Check sheet for the modelled part. Datum: model origin and axes. Units: mm. Face numbers are marked on the shaded views. A direction names the side the tool comes from. Give positions to 0.01 mm unless a question says otherwise; leave off trailing zeros. Order: outer loops, then holes, each group sorted by start corner. A loop starts at its lowest first (then second) coordinate and runs counter-clockwise, first axis right, second up. Notation, with made-up numbers: (18.5, -18.75) -> (69.5, -18.75) arc R10 cw to (69.5, -10.75) -> close; hole circle Ø9 at (58, 17). An arc over 180 degrees is marked (long way). Write each question's results on one line, items separated by ' | '.
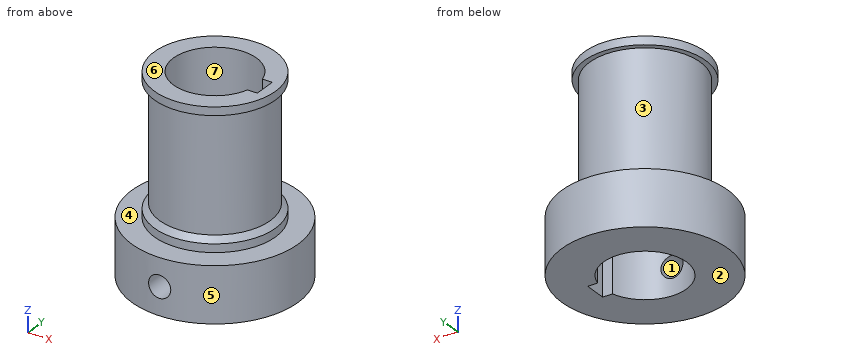
from build123d import *

# Parameters (mm, degrees)
F0_R      = 30
F1_DEPTH  = 20
F3_R      = 21.9
F4_DEPTH  = 3
F6_R      = 21.9
F7_DEPTH  = 2
F9_R      = 20
F10_DEPTH = 42
F11_SIZE2 = 1.99999
F11_SIZE  = 1.89999
F12_R     = 21.9
F13_DEPTH = 3
F15_DEPTH = 78
F16_R     = 4
F17_DEPTH = 45


# Not quite as in the source:
# - a fillet or chamfer is up to 0.001 mm smaller than in the source, because OpenCascade refuses the exact size


with BuildPart() as f1:
    # F0 (on Top) → F1 (new body)
    with BuildSketch(Plane.XY):
        Circle(F0_R)
    extrude(amount=F1_DEPTH)

    # F3 (on offset) → F4 (join)
    with BuildSketch(Plane.XY.offset(20)):
        Circle(F3_R)
    extrude(amount=F4_DEPTH)

    # F6 (on offset) → F7 (join)
    with BuildSketch(Plane.XY.offset(23)):
        Circle(F6_R)
    extrude(amount=F7_DEPTH)

    # F9 (on offset) → F10 (join)
    with BuildSketch(Plane.XY.offset(25)):
        Circle(F9_R)
    extrude(amount=F10_DEPTH)

    # F11 (size 1.9 and 2 in the source; OpenCascade refuses exactly that, so slightly less here)
    f11_edges = [f1.edges().sort_by_distance(p)[0] for p in [
        (-21.9, 0, 25),
    ]]
    f11_side = f1.faces().sort_by_distance((-21.280574, 0, 25))[0]
    chamfer(f11_edges, length=F11_SIZE, length2=F11_SIZE2, reference=f11_side)

    # F12 (on face) → F13 (join)
    with BuildSketch(Plane.XY.offset(67)):
        Circle(F12_R)
    extrude(amount=F13_DEPTH)

    # F14 (on face) → F15 (cut)
    with BuildSketch(Plane.XY.offset(70)):
        with BuildLine():
            Line((18, 4), (14.4568322948, 4))
            ThreePointArc((14.4568322948, 4), (-15, 0), (14.4568322948, -4))
            Line((14.4568322948, -4), (18, -4))
            Line((18, -4), (18, 0))
            Line((18, 0), (18, 4))
        make_face()
    extrude(amount=-F15_DEPTH, mode=Mode.SUBTRACT)

    # F16 (on Front) → F17 (cut)
    with BuildSketch(Plane.XZ):
        with Locations((0, 10)):
            Circle(F16_R)
    extrude(amount=F17_DEPTH, mode=Mode.SUBTRACT)


solid = f1.part
1. Gauge pin test, flat ends, axial feed: pin 1 Ø1.8 at (x, z) = (16.5, 52) entering from +Y; pin 2 Ø10 at (y, z) = (2.5, 58.5) entering from -X; pin 3 Ø7 at (x, z) = (0, 10) entering from -Y; pin 4 Ø24 at (x, y) = (0, 0) entering from +Z. Record the tip position at first contact, or that the pin passes through.
Verdict:
pin 1: stops at y = 12.52 | pin 2: stops at x = -20 | pin 3: stops at y = 14.59 | pin 4: passes through
2. Material ranges on probe 1 along Z at (x, y) = (0, -22); probe 2 along Y at (x, z) = (0, 23); probe 3 along Y at (x, z) = (0, 33), recorded low to high. Write a range as from..to.
Verdict:
probe 1: z = 0..6, 14..20 | probe 2: y = -21.9..-15, 15..21.9 | probe 3: y = -20..-15, 15..20
3. Section check C-C on z = 18.5. Record the cut outline in (x, y), then the cut area to 3 significant figures.
Verdict:
outline: circle Ø60 at (0, 0); hole (14.46, -4) -> (18, -4) -> (18, 4) -> (14.46, 4) arc R15 ccw (long way) to start | area: 2,100 mm^2
4. Section check D-D on y = -25.5. Record the cut outline in (x, z).
Verdict:
outline: (-15.8, 0) -> (15.8, 0) -> (15.8, 20) -> (-15.8, 20) -> close; hole circle Ø8 at (0, 10)
5. Mould release check, pull along X, two halves, no side actions. Record for the marked faces 5, 6 and 7: +X half, -X half, draft (parallel to the pull), parting line (faces both ways), or undercut.
Verdict:
face 5: parting line | face 6: draft | face 7: undercut
6. Section check B-B on x = 0. Give the number of separate pieces and of enclosed holes in the cut face, then the cut area to 3 significant figures.
Verdict:
separate pieces: 3 | enclosed holes: 0 | area: 1,010 mm^2
7. Access from +Z, -Z, +X, -X, +Y, -Y to the whole of each face (thin tool, end or side, straight path). Record for the marked faces 1, 2, 3 and 4.
Verdict:
face 1: -Y | face 2: -Z, +X, -X, +Y, -Y | face 3: none | face 4: +Z
